The drawing under review shows one solid part. Ordinate dimensions are in mm from its lowest x, y, z. A direction names the side the tool comes from. Coordinates: 2 decimals unless noted, no trailing zeros. Write each loop counter-clockwise with the first axis right and the second up, starting at its lowest first coordinate (ties: lowest second). Pieces come first, ordered by that corner, then holes.
Q1. For probe 1 along Y at (x, z) = (10, 19.55); probe 2 along Z at (x, y) = (0.45, 15); probe 3 along Z at (x, y) = (0.3, 10), list the stretches that pass through material, from the lowest coordinate up.
Q2. Take a section at B-B (x = 16.25). Give the boundary of the cut face in (y, z), and give its area (3 significant figures).
Q3. Insertion check: pin 1 (2.5 mm diameter, centred on x = 5, z = 16, fed in from -Y); pin 2 (12 mm diameter, centred on x = 9, y = 5, fed in from +Z); pin 3 (4.5 mm diameter, centred on x = 5, z = 15, fed in from +Y); pin 4 (4.5 mm diameter, centred on y = 15, z = 5, fed in from -X). Each pin has a flat end and moves straight along its axis. Give the tip position at first contact, or say it passes through.
Q4. Take a section at C-C (y = 12). Give the boundary of the cut face in (x, z).
Q5. Take a section at D-D (z = 10). Give the boundary of the cut face in (x, y), and give its area (3 significant figures).
Q6. Take a section at A-A (z = 16). Give the boundary of the cut face in (x, y), and give its area (3 significant figures).
Q7. Mouldability with a two-part tool opening along Y and no side actions: class the marked faces 6, 7, 8 and 9 as pulls with the +Y half, pulls with the -Y half, needs draft (parallel to the pull), parting line crosses it, or undercut.
Q8. Machinability: for the marked faces 1, 2, 3, 4 and 5, which of the approach directions +Z, -Z, +X, -X, +Y, -Y give a long, thin tool a straight path to every point of the face, cutting with its end or side? Answer none if there is none.
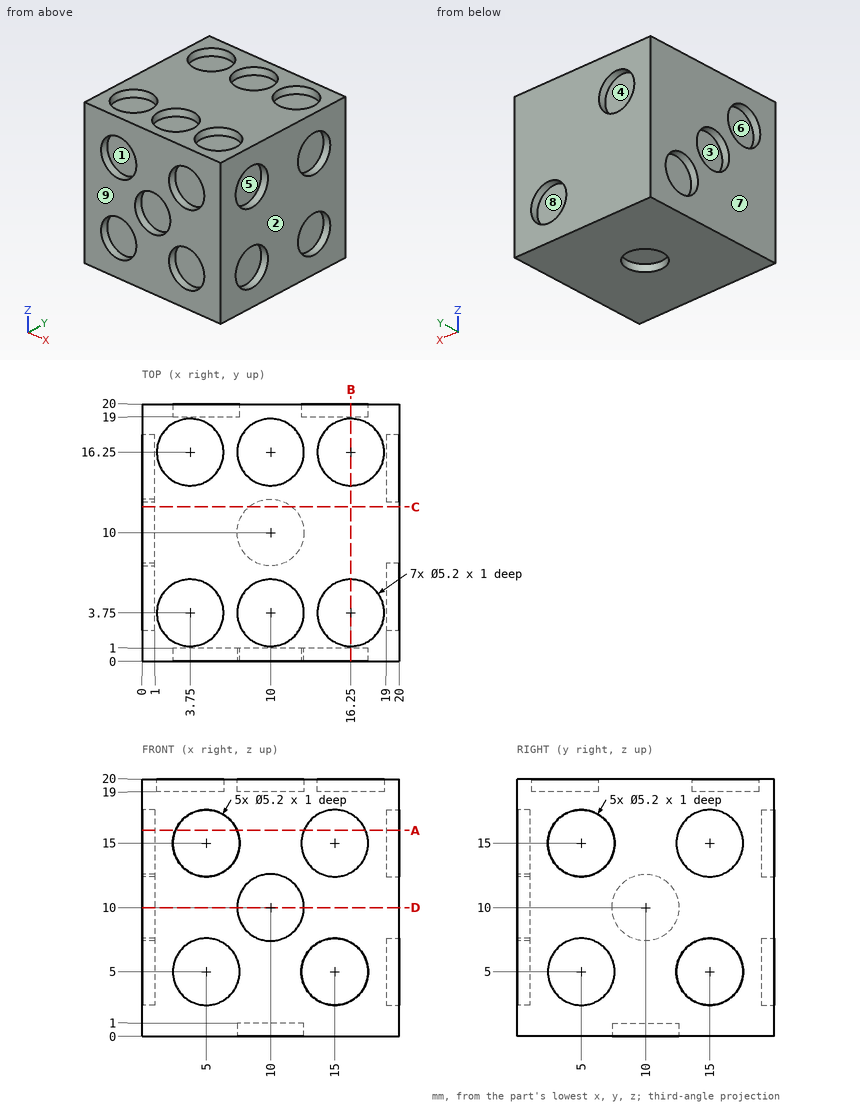
Response:
1. probe 1: y = 0 to 1.15, 6.35 to 13.65, 18.85 to 20
1. probe 2: z = 0 to 2.4, 7.6 to 20
1. probe 3: z = 0 to 7.4, 12.6 to 20
2. outline: (0, 0) - (20, 0) - (20, 2.72) - (19, 2.72) - (19, 7.28) - (20, 7.28) - (20, 20) - (18.85, 20) - (18.85, 19) - (13.65, 19) - (13.65, 20) - (6.35, 20) - (6.35, 19) - (1.15, 19) - (1.15, 20) - (0, 20) - (0, 17.28) - (1, 17.28) - (1, 12.72) - (0, 12.72) - (0, 7.28) - (1, 7.28) - (1, 2.72) - (0, 2.72) - close
2. area: 376 mm2
3. pin 1: stops at y = 1
3. pin 2: stops at z = 20
3. pin 3: stops at y = 19
3. pin 4: stops at x = 1
4. outline: (0, 0) - (8.34, 0) - (8.34, 1) - (11.66, 1) - (11.66, 0) - (20, 0) - (20, 20) - (0, 20) - (0, 11.66) - (1, 11.66) - (1, 8.34) - (0, 8.34) - close
5. outline: (0, 0) - (7.4, 0) - (7.4, 1) - (12.6, 1) - (12.6, 0) - (20, 0) - (20, 20) - (0, 20) - (0, 12.6) - (1, 12.6) - (1, 7.4) - (0, 7.4) - close
5. area: 390 mm2
6. outline: (0, 0) - (2.6, 0) - (2.6, 1) - (7.4, 1) - (7.4, 0) - (12.6, 0) - (12.6, 1) - (17.4, 1) - (17.4, 0) - (20, 0) - (20, 2.6) - (19, 2.6) - (19, 7.4) - (20, 7.4) - (20, 12.6) - (19, 12.6) - (19, 17.4) - (20, 17.4) - (20, 20) - (7.4, 20) - (7.4, 19) - (2.6, 19) - (2.6, 20) - (0, 20) - (0, 7.4) - (1, 7.4) - (1, 2.6) - (0, 2.6) - close
6. area: 371 mm2
7. face 6: undercut
7. face 7: needs draft
7. face 8: pulls with the +Y half
7. face 9: pulls with the -Y half
8. face 1: -Y
8. face 2: +Z, -Z, +X, +Y, -Y
8. face 3: -X
8. face 4: +Y
8. face 5: +X
